Input: part model. Units: mm. Frame: model coordinates. A direction names the side the tool comes from. Round coordinates to 2 decimals unless told otherwise and drop trailing zeros. Order: outer loops, then holes, each group sorted by start corner. A loop starts at its lowest first (then second) coordinate and runs counter-clockwise, first axis right, second up. Notation, with made-up numbers: M -32,-36.5 L 18,-36.5 A15 ccw 18,-31.5 Z; hole C -2.75,23 d11. An arc over 180 degrees is marked long. One line per question, with ' | ' between items.
```python
from build123d import *

# Parameters (mm, degrees)
F1_W      = 50.8
F1_H      = 50.8
F1_W_2    = 44.45
F1_H_2    = 44.45
F2_DEPTH  = 304.8
F4_DEPTH  = 50.801
F6_DEPTH  = 127
F7_R      = 14.2875
F8_DEPTH  = 50.801
F9_W      = 76.2
F9_H      = 25.4
F10_DEPTH = 50.801
F11_R     = 19.05
F12_DEPTH = 50.8


with BuildPart() as f2:
    # F1 (on face) → F2 (new body)
    with BuildSketch(Plane.XZ):
        Rectangle(F1_W, F1_H)
        Rectangle(F1_W_2, F1_H_2, mode=Mode.SUBTRACT)
    extrude(amount=F2_DEPTH)

    # F3 (on face) → F4 (cut, through all)
    with BuildSketch(Plane.YZ.offset(25.4)):
        Polygon((-283.757951, 25.4), (-304.8, 25.4), (-304.8, -25.4), align=None)
    extrude(amount=-F4_DEPTH, mode=Mode.SUBTRACT)

    # F5 (on face) → F6 (cut)
    with BuildSketch(Plane.YZ.offset(25.4)):
        Polygon((0, -25.4), (0, 25.4), (-21.042049, 25.4), align=None)
    extrude(amount=-F6_DEPTH, mode=Mode.SUBTRACT)

    # F7 (on face) → F8 (cut, through all)
    with BuildSketch(Plane.XY.offset(25.4)):
        with Locations((0, -152.4)):
            Circle(F7_R)
    extrude(amount=-F8_DEPTH, mode=Mode.SUBTRACT)

    # F9 (on face) → F10 (cut, through all)
    with BuildSketch(Plane(origin=(-25.4, 0, 0), x_dir=(0, -1, 0), z_dir=(-1, 0, 0))):
        with Locations((152.4, 0)):
            Rectangle(F9_W, F9_H)
    extrude(amount=-F10_DEPTH, mode=Mode.SUBTRACT)

    # F11 (on face) → F12 (cut)
    with BuildSketch(Plane.XY.offset(25.4)):
        with Locations((0, -252.007951)):
            Circle(F11_R)
        with Locations((0, -201.207951)):
            Circle(F11_R)
        with Locations((0, -103.592049)):
            Circle(F11_R)
        with Locations((0, -52.792049)):
            Circle(F11_R)
    extrude(amount=-F12_DEPTH, mode=Mode.SUBTRACT)


solid = f2.part
```
Item 1: Section query A-A, the plane y = -152.4. Return loops of the section in (x, z) (1 decimal).
Report:
outline: M -25.4,-25.4 L -14.3,-25.4 L -14.3,-22.2 L -22.2,-22.2 L -22.2,-12.7 L -25.4,-12.7 Z; M -25.4,12.7 L -22.2,12.7 L -22.2,22.2 L -14.3,22.2 L -14.3,25.4 L -25.4,25.4 Z; M 14.3,-25.4 L 25.4,-25.4 L 25.4,-12.7 L 22.2,-12.7 L 22.2,-22.2 L 14.3,-22.2 Z; M 14.3,22.2 L 22.2,22.2 L 22.2,12.7 L 25.4,12.7 L 25.4,25.4 L 14.3,25.4 Z
Item 2: Line query: line 1 along Y through (x, z) = (0, -23.85); line 2 along Y through (x, z) = (0, 23.85); line 3 along Z through (x, y) = (-9.5, -276) (3 decimals). Output: solid intervals per line, ascending. Write a range as from..to.
Report:
line 1: -304.16..-271.06, -232.96..-220.26, -182.16..-166.69, -138.11..-122.64, -84.54..-71.84, -33.74..-0.64 | line 2: -284.4..-271.06, -232.96..-220.26, -182.16..-166.69, -138.11..-122.64, -84.54..-71.84, -33.74..-20.4 | line 3: -25.4..-22.225, 22.225..25.4
Item 3: First-contact query: pin 1 (17 mm diameter, centred on x = 0, y = -152.4, fed in from -Z). Flat tip, straight axial feed; report the tip coordinate or a pass-through.
Report:
pin 1: through
Item 4: Access query for faces 5 (the flat face through (17, -150, -25.4)), 6 (the flat face through (-22.225, -150, -15)). Directions: +Z, -Z, +X, -X, +Y, -Y. A direction counts if a zero-diameter tool reaches every point of the face in a straight line with its end or side. Return the directions, or none.
Report:
face 5: -Z, +X, -X, +Y, -Y | face 6: +Y, -Y
Item 5: Mould query, pull axis Z, two halves, no side actions, for faces 1 (the flat face through (-17, -151, 25.4)), 2 (the cylindrical face through (-4.13, -219.805, -23.79)), 3 (the flat face through (-15, -150, -22.225)), 4 (the flat face through (22.225, -150, -15)). Classes: +Z half, -Z half, draft (parallel to the pull), parting line (faces both ways), or undercut.
Report:
face 1: +Z half | face 2: draft | face 3: undercut | face 4: undercut
Item 6: Section query C-C, the plane y = -209. Return loops of the section in (x, z) (3 decimals).
Report:
outline: M -25.4,-25.4 L -17.384,-25.4 L -17.384,-22.225 L -22.225,-22.225 L -22.225,22.225 L -17.384,22.225 L -17.384,25.4 L -25.4,25.4 Z; M 17.384,-25.4 L 25.4,-25.4 L 25.4,25.4 L 17.384,25.4 L 17.384,22.225 L 22.225,22.225 L 22.225,-22.225 L 17.384,-22.225 Z
Item 7: Section query B-B, the plane x = 0. Give the number of separate pieces and of enclosed holes in the cut face, plus the area to 3 significant figures.
Report:
separate pieces: 12 | enclosed holes: 0 | area: 653 mm²
